Read the model definition and answer for the solid it produces. Units are mm, in the model's axes. Face numbers are marked on the shaded views. A direction names the side the tool comes from. Give positions to 0.01 mm unless a question says otherwise; leave off trailing zeros. Write each loop counter-clockwise with the first axis right and the second up, starting at its lowest first coordinate (ties: lowest second). Pieces come first, ordered by that corner, then holes.
```python
from build123d import *

# Parameters (mm, degrees)
F0_W     = 76.2
F0_H     = 50.8
F0_R     = 12.7
F1_DEPTH = 12.7
F2_W     = 6.35
F2_H     = 50.8
F3_DEPTH = 15.24
F5_DEPTH = 50.8


with BuildPart() as f1:
    # F0 (on Top) → F1 (new body)
    with BuildSketch(Plane.XY):
        Rectangle(F0_W, F0_H)
        Circle(F0_R, mode=Mode.SUBTRACT)
    extrude(amount=F1_DEPTH)

    # F2 (on face) → F3 (join)
    with BuildSketch(Plane.XY.offset(12.7)):
        with Locations((-32.385, 0)):
            Rectangle(F2_W, F2_H)
        with BuildLine():
            Line((-6.35, -10.998523), (-6.35, -25.4))
            Line((-6.35, -25.4), (6.35, -25.4))
            Line((6.35, -25.4), (6.35, -10.998523))
            ThreePointArc((6.35, -10.998523), (0, -12.7), (-6.35, -10.998523))
        make_face()
        with BuildLine():
            Line((6.35, 25.4), (-6.35, 25.4))
            Line((-6.35, 25.4), (-6.35, 10.998523))
            ThreePointArc((-6.35, 10.998523), (0, 12.7), (6.35, 10.998523))
            Line((6.35, 10.998523), (6.35, 25.4))
        make_face()
    extrude(amount=-F3_DEPTH)

    # F4 (on face) → F5 (join)
    with BuildSketch(Plane.XZ.offset(25.4)):
        Polygon((31.75, 0), (19.05, 0), (16.117061, -5.08), (34.682939, -5.08), align=None)
    extrude(amount=-F5_DEPTH)


solid = f1.part
```
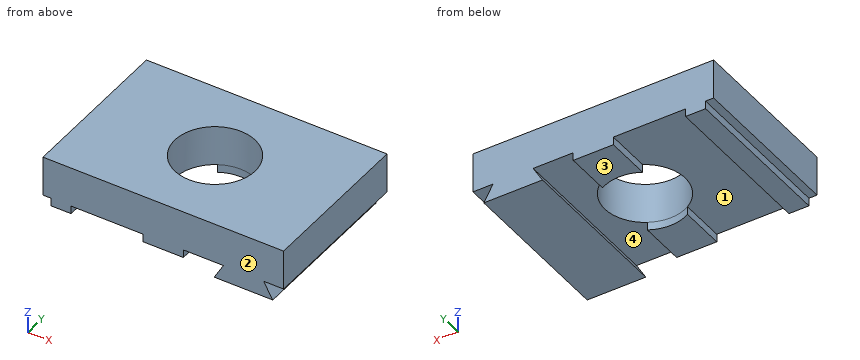
Item 1: Which of the six approach directions +Z, -Z, +X, -X, +Y, -Y give full straight-line access (tool end or side, diameter ignored) to the marked faces 1, 2, 3 and 4?
Result set:
face 1: -Z, +Y, -Y
face 2: +Z, -Z, +X, -X, -Y
face 3: -Z, -X, +Y, -Y
face 4: +Y, -Y
Item 2: Section D-D (z = 5.5) is taken. Write down the section's boundary in (x, y).
Result set:
outline: (-38.1, -25.4) - (38.1, -25.4) - (38.1, 25.4) - (-38.1, 25.4) - close; hole circle Ø25.4 at (0, 0)
Item 3: Each of these flat-tipped pins is pushed along its axis until it touches: pin 1 Ø8 at (x, y) = (-20, 16) entering from -Z; pin 2 Ø1.5 at (x, y) = (0.5, -13) entering from -Z; pin 3 Ø0.8 at (y, z) = (-21.5, -1) entering from +X; pin 4 Ø2 at (y, z) = (-20.5, -0.5) entering from -X. Where does it stop, or does it pass through?
Result set:
pin 1: stops at z = 0
pin 2: stops at z = -2.54
pin 3: stops at x = 32.56
pin 4: stops at x = -38.1
Item 4: Section A-A (x = 0) is taken. Write down the section's boundary in (y, z), and give its area (3 significant figures).
Result set:
outline: (-25.4, -2.54) - (-12.7, -2.54) - (-12.7, 12.7) - (-25.4, 12.7) - close; (12.7, -2.54) - (25.4, -2.54) - (25.4, 12.7) - (12.7, 12.7) - close
area: 387 mm2
Item 5: Find the intervals of material crossed by line 1 along X through (y, z) = (0, 8); line 2 along Y through (x, z) = (0.5, -2); line 3 along Z through (x, y) = (-18.5, 5), in increasing order.
Result set:
line 1: x = -38.1 to -12.7, 12.7 to 38.1
line 2: y = -25.4 to -12.69, 12.69 to 25.4
line 3: z = 0 to 12.7
Item 6: Section B-B (y = 0) is taken. Write down the section's boundary in (x, z).
Result set:
outline: (-38.1, 0) - (-35.56, 0) - (-35.56, -2.54) - (-29.21, -2.54) - (-29.21, 0) - (-12.7, 0) - (-12.7, 12.7) - (-38.1, 12.7) - close; (12.7, 0) - (19.05, 0) - (16.12, -5.08) - (34.68, -5.08) - (31.75, 0) - (38.1, 0) - (38.1, 12.7) - (12.7, 12.7) - close
Item 7: Section C-C (y = 20.5) is taken. Write down the section's boundary in (x, z).
Result set:
outline: (-38.1, 0) - (-35.56, 0) - (-35.56, -2.54) - (-29.21, -2.54) - (-29.21, 0) - (-6.35, 0) - (-6.35, -2.54) - (6.35, -2.54) - (6.35, 0) - (19.05, 0) - (16.12, -5.08) - (34.68, -5.08) - (31.75, 0) - (38.1, 0) - (38.1, 12.7) - (-38.1, 12.7) - close
